```python
from build123d import *

# Parameters (mm, degrees)
F0_R     = 1.5875
F1_DEPTH = 3.048


with BuildPart() as f1:
    # F0 (on Front) → F1 (new body)
    with BuildSketch(Plane.XZ):
        with BuildLine():
            ThreePointArc((9.48492, 113.427124), (9.514975, 113.863102), (9.525, 114.3))
            ThreePointArc((9.525, 114.3), (0.060685, 123.824807), (-9.524227, 114.421367))
            ThreePointArc((-9.524227, 114.421367), (-0.497509, 104.788002), (9.48492, 113.427124))
        make_face()
        with BuildLine():
            ThreePointArc((9.48492, 113.427124), (-0.497509, 104.788002), (-9.524227, 114.421367))
            Line((-9.524227, 114.421367), (-15.489332, 60.627964))
            ThreePointArc((-15.489332, 60.627964), (-0.379702, 73.020458), (15.305283, 61.364727))
            Line((15.305283, 61.364727), (9.48492, 113.427124))
        make_face()
        with Locations((0, 95.112495)):
            Circle(F0_R, mode=Mode.SUBTRACT)
        with BuildLine():
            Line((-15.875, 57.15), (-15.489332, 60.627964))
            ThreePointArc((-15.489332, 60.627964), (-15.778288, 58.899641), (-15.875, 57.15))
        make_face()
        with BuildLine():
            ThreePointArc((15.305283, 61.364727), (-0.379702, 73.020458), (-15.489332, 60.627964))
            Line((-15.489332, 60.627964), (-15.875, 57.15))
            Line((-15.875, 57.15), (-15.285187, 52.862963))
            ThreePointArc((-15.285187, 52.862963), (-0.943722, 41.303076), (14.668351, 51.07916))
            Line((14.668351, 51.07916), (15.734881, 59.25455))
            ThreePointArc((15.734881, 59.25455), (15.555905, 60.316931), (15.305283, 61.364727))
        make_face()
        with BuildLine():
            Line((-15.285187, 52.862963), (-15.875, 57.15))
            ThreePointArc((-15.875, 57.15), (-15.726856, 54.98629), (-15.285187, 52.862963))
        make_face()
        with BuildLine():
            ThreePointArc((15.875, 57.15), (15.839932, 58.204605), (15.734881, 59.25455))
            Line((15.734881, 59.25455), (14.668351, 51.07916))
            ThreePointArc((14.668351, 51.07916), (15.570416, 54.055202), (15.875, 57.15))
        make_face()
        with BuildLine():
            ThreePointArc((14.668351, 51.07916), (-0.943722, 41.303076), (-15.285187, 52.862963))
            Line((-15.285187, 52.862963), (-7.863428, -1.081855))
            ThreePointArc((-7.863428, -1.081855), (-0.542194, 7.91896), (7.9375, 0))
            ThreePointArc((7.9375, 0), (6.707453, -4.244288), (3.398545, -7.17313))
            Line((3.398545, -7.17313), (41.051455, -7.17313))
            ThreePointArc((41.051455, -7.17313), (36.604764, -1.20672), (39.052875, 5.820219))
            Line((39.052875, 5.820219), (17.676814, 6.4068))
            ThreePointArc((17.676814, 6.4068), (11.849313, 9.191003), (10.011494, 15.382447))
            Line((10.011494, 15.382447), (14.668351, 51.07916))
        make_face()
        with BuildLine():
            ThreePointArc((7.9375, 0), (-0.542194, 7.91896), (-7.863428, -1.081855))
            ThreePointArc((-7.863428, -1.081855), (-3.776202, -6.981705), (3.398545, -7.17313))
            ThreePointArc((3.398545, -7.17313), (6.707453, -4.244288), (7.9375, 0))
        make_face()
        with BuildLine():
            ThreePointArc((39.052875, 5.820219), (36.604764, -1.20672), (41.051455, -7.17313))
            ThreePointArc((41.051455, -7.17313), (48.694288, -6.707453), (52.3875, 0))
            ThreePointArc((52.3875, 0), (47.625234, 7.274737), (39.052875, 5.820219))
        make_face()
    extrude(amount=F1_DEPTH)


solid = f1.part
```
The model under review builds one solid part; all positions refer to its coordinate system, in mm. A direction names the side the tool comes from. Coordinates: 2 decimals unless noted, no trailing zeros. Write each loop counter-clockwise with the first axis right and the second up, starting at its lowest first coordinate (ties: lowest second). Pieces come first, ordered by that corner, then holes. Notation, with made-up numbers: (24.5, 63.5) - (62.5, 63.5) arc R7 ccw to (62.5, 76.5) - close; hole circle Ø5 at (-36, 70.5). An arc over 180 degrees is marked (long way). Answer in a Markdown table with one row per item. Add a question column.
Q1. Draft analysis for pull direction X (two halves, no side actions). For faces 4 (the face through (-12.465, -1.503, 87.901)), 5 (the face through (3, -3.048, 44)), 6 (the face through (-3.87, -1.5, -6.93)), state which applies: +X half, -X half, draft (parallel to the pull), parting line (faces both ways), or undercut.
Q2. Consider section D-D on x = 34. Give the boundary of the cut face in (y, z).
Q3. For faces 1 (the face through (11.91, -1.5, 9.12)), 2 (the face through (15.56, -1.5, 54.01)), 3 (the face through (22, -2, -7.173)), list the 3-axis set-ups (+Z, -Z, +X, -X, +Y, -Y) from which the entire face can be reached by the end or side of a thin tool; tool diameter is ignored.
Q4. To check wall thickness, follow line 1 along Z through (x, y) = (0, -2.4) (1 decimal); line 2 along Z through (x, y) = (18.5, -2.65); line 3 along X through (y, z) = (-2, 68). State the ranges of each line that lie inside material, in increasing order. Write a range as from..to.
Q5. Consider section C-C on z = 74.5. Give the boundary of the cut face in (x, y).
Q6. Clearance check with flat-ended pins moving along their axes: pin 1 (1.5 mm diameter, centred on x = 17.5, y = -1.5, fed in from -Z); pin 2 (1 mm diameter, centred on y = -2.5, z = 53, fed in from -X). State where each tip first meets the part, or that it passes through.
Q7. Consider section A-A on x = 0. Give the boundary of the cut face in (y, z) (1 decimal).
Answers below:
| question | item | result |
|---|---|---|
| 1 | face 4 | -X half |
| 1 | face 5 | draft |
| 1 | face 6 | undercut |
| 2 | outline | (-3.05, -7.17) - (0, -7.17) - (0, 5.96) - (-3.05, 5.96) - close |
| 3 | face 1 | +Y, -Y |
| 3 | face 2 | +X, +Y, -Y |
| 3 | face 3 | -Z, +Y, -Y |
| 4 | line 1 | -7.9..93.5, 96.7..123.8 |
| 4 | line 2 | -7.17..6.38 |
| 4 | line 3 | -14.67..14.56 |
| 5 | outline | (-13.95, -3.05) - (13.84, -3.05) - (13.84, 0) - (-13.95, 0) - close |
| 6 | pin 1 | z = -7.17 |
| 6 | pin 2 | x = -15.45 |
| 7 | outline | (-3, -7.9) - (0, -7.9) - (0, 93.5) - (-3, 93.5) - close; (-3, 96.7) - (0, 96.7) - (0, 123.8) - (-3, 123.8) - close |
